Can you work these out from the model? Positions are in its coordinate system, mm. A direction names the side the tool comes from. Coordinates: 2 decimals unless noted, no trailing zeros. Loops run counter-clockwise (first coordinate to the right, second up) from the corner with the lowest first, then second, coordinate; pieces in that order, holes last.
```python
from build123d import *

# Parameters (mm, degrees)
F0_W     = 60
F0_H     = 70
F1_DEPTH = 25
F2_R     = 10
F3_DEPTH = 25
F4_R     = 7.5
F4_R_2   = 0.5
F5_DEPTH = 10


with BuildPart() as f1:
    # F0 (on Top) → F1 (new body)
    with BuildSketch(Plane.XY):
        Rectangle(F0_W, F0_H)
        Polygon((18, 33), (28, 23), (28, -23), (18, -33), (-18, -33), (-28, -23), (-28, 23), (-18, 33), align=None, mode=Mode.SUBTRACT)
    extrude(amount=F1_DEPTH)

    # F2 (on face) → F3 (join)
    with BuildSketch(Plane.XZ.offset(35)):
        with Locations((0, 12.5)):
            Circle(F2_R)
    extrude(amount=F3_DEPTH)

    # F4 (on face) → F5 (join)
    with BuildSketch(Plane(origin=(0, 35, 0), x_dir=(-1, 0, 0), z_dir=(0, 1, 0))):
        with Locations((0, 12.5)):
            Circle(F4_R)
        with Locations((0, 12.5)):
            Circle(F4_R_2, mode=Mode.SUBTRACT)
    extrude(amount=F5_DEPTH)


solid = f1.part
```
(1) I'm going to push flat-ended pins straight in: pin 1 (8 mm diameter, centred on x = 9.5, z = 3, fed in from +Y); pin 2 (1 mm diameter, centred on y = -37.5, z = 10.5, fed in from -X); pin 3 (5 mm diameter, centred on x = 12.5, z = 17.5, fed in from -Y). Where does each tip first touch, or does it pass through?
Check values:
pin 1: stops at y = 35
pin 2: stops at x = -9.89
pin 3: stops at y = -35
(2) I want a section at A-A on z = 18.5. Write out the boundary of the cut face in (x, y), then the cut area to 3 significant figures.
Check values:
outline: (-30, -35) - (-8, -35) - (-8, -60) - (8, -60) - (8, -35) - (30, -35) - (30, 35) - (4.5, 35) - (4.5, 45) - (-4.5, 45) - (-4.5, 35) - (-30, 35) - close; hole (-28, -23) - (-18, -33) - (18, -33) - (28, -23) - (28, 23) - (18, 33) - (-18, 33) - (-28, 23) - close
area: 1,190 mm2
(3) Which directions (+Z, -Z, +X, -X, +Y, -Y) give clear straight access to the entire face, cutting with the end or side of a thin tool? Please do faces 4 (the cylindrical face through (-2.17, -47.32, 2.74)), 5 (the flat face through (-7.1, 35, 9.5)), 6 (the flat face through (-23, 28, 12)).
Check values:
face 4: -Y
face 5: +Y
face 6: +Z, -Z
(4) I want a section at B-B on x = -26. Write out the boundary of the cut face in (y, z).
Check values:
outline: (-35, 0) - (-25, 0) - (-25, 25) - (-35, 25) - close; (25, 0) - (35, 0) - (35, 25) - (25, 25) - close
(5) I want a section at C-C on y = -13.5. Write out the boundary of the cut face in (x, z).
Check values:
outline: (-30, 0) - (-28, 0) - (-28, 25) - (-30, 25) - close; (28, 0) - (30, 0) - (30, 25) - (28, 25) - close
(6) I want a section at D-D on y = 39.5. Write out the boundary of the cut face in (x, z), then the cut area to 3 significant figures.
Check values:
outline: circle Ø15 at (0, 12.5); hole circle Ø1 at (0, 12.5)
area: 176 mm2
(7) If we mould it in two halves opening along X, with no side actions, what happens to faces 1 (the cylindrical face through (1.63, 39.93, 5.18)), 2 (the flat face through (-29, 0, 25)), 3 (the flat face through (23, 28, 12))? For each: released by +X, released by -X, zero draft, split by the parting line, or undercut.
Check values:
face 1: split by the parting line
face 2: zero draft
face 3: undercut
(8) If I drill on probe 1 along Z at (x, y) = (0, 39); probe 2 along Y at (x, z) = (-15, 14); probe 3 along Y at (x, z) = (3, 12.25), over which ranges is the centre line in solid material (lowest first)?
Check values:
probe 1: z = 5 to 12, 13 to 20
probe 2: y = -35 to -33, 33 to 35
probe 3: y = -60 to -33, 33 to 45
